```python
from build123d import *

# Parameters (mm, degrees)
BOSS_EXTRUDE1_START     = -12.7
BOSS_EXTRUDE1_OUTLINE_R = 9.525
BOSS_EXTRUDE1_DEPTH     = 12.7
SKETCH1_R               = 7.9375
BOSS_EXTRUDE2_DEPTH     = 127
BOSS_EXTRUDE3_START     = 25.4
SKETCH2_R               = 9.525
BOSS_EXTRUDE3_DEPTH     = 25.4
CHAMFER2_SIZE           = 1.5875
CUT_EXTRUDE1_DEPTH      = 166.648607751
CUT_EXTRUDE1_DEPTH_BACK = 166.648607751
SKETCH3_R               = 4.7625


# Read off the part's stored shape, not the designer's step: Boss-Extrude1
with BuildPart() as part:
    # Boss-Extrude1 outline → Boss-Extrude1 (new body)
    with BuildSketch(Plane.XY.offset(BOSS_EXTRUDE1_START)):
        Circle(BOSS_EXTRUDE1_OUTLINE_R)
    extrude(amount=BOSS_EXTRUDE1_DEPTH)

    # Sketch1 → Boss-Extrude2 (add)
    with BuildSketch(Plane(origin=(0, 0, -12.7), x_dir=(-1, 0, 0), z_dir=(0, 0, -1))):
        Circle(SKETCH1_R)
    extrude(amount=BOSS_EXTRUDE2_DEPTH)

    # Sketch2 → Boss-Extrude3 (add)
    with BuildSketch(Plane(origin=(0, 0, -139.7), x_dir=(-1, 0, 0), z_dir=(0, 0, -1)).offset(BOSS_EXTRUDE3_START)):
        Circle(SKETCH2_R)
    extrude(amount=-BOSS_EXTRUDE3_DEPTH)

    # Chamfer2
    chamfer2_edges = [part.edges().sort_by_distance(p)[0] for p in [
        (9.525, 0, -165.1),
    ]]
    chamfer(chamfer2_edges, length=CHAMFER2_SIZE)

    # Sketch3 → Cut-Extrude1 (cut, two sides: drawn at the far end of the back side and taken through both)
    with BuildSketch(Plane(origin=(0, 0, 0), x_dir=(0, 0, -1), z_dir=(1, 0, 0)).offset(-CUT_EXTRUDE1_DEPTH_BACK)):
        with Locations((152.4, 0)):
            Circle(SKETCH3_R)
    extrude(amount=CUT_EXTRUDE1_DEPTH + CUT_EXTRUDE1_DEPTH_BACK, mode=Mode.SUBTRACT)


solid = part.part
```
For this review, take the finished solid that the model builds, in its own axes (mm). A direction names the side the tool comes from. Round coordinates to 2 decimals unless told otherwise and drop trailing zeros. Write each loop counter-clockwise with the first axis right and the second up, starting at its lowest first coordinate (ties: lowest second). Pieces come first, ordered by that corner, then holes. Notation, with made-up numbers: (-7.5, 53.5) - (31.5, 53.5) arc R28 cw to (31.5, 88.5) - close; hole circle Ø4 at (8.5, 61.25). An arc over 180 degrees is marked (long way). Put each result on its own line as item: value.
Q1. We need section B-B (x = 0). Give the boundary of the cut face in (y, z) (1 decimal).
Solved:
outline: (-9.5, -163.5) - (-7.9, -165.1) - (7.9, -165.1) - (9.5, -163.5) - (9.5, -139.7) - (7.9, -139.7) - (7.9, -12.7) - (9.5, -12.7) - (9.5, 0) - (-9.5, 0) - (-9.5, -12.7) - (-7.9, -12.7) - (-7.9, -139.7) - (-9.5, -139.7) - close; hole circle Ø9.5 at (0, -152.4)
Q2. We need section A-A (y = 0). Give the boundary of the cut face in (x, z) (1 decimal), and give its area (3 significant figures).
Solved:
outline: (-9.5, -163.5) - (-7.9, -165.1) - (7.9, -165.1) - (9.5, -163.5) - (9.5, -157.2) - (-9.5, -157.2) - close; (-9.5, -147.6) - (9.5, -147.6) - (9.5, -139.7) - (7.9, -139.7) - (7.9, -12.7) - (9.5, -12.7) - (9.5, 0) - (-9.5, 0) - (-9.5, -12.7) - (-7.9, -12.7) - (-7.9, -139.7) - (-9.5, -139.7) - close
area: 2,560 mm2
Q3. Insertion check: pin 1 Ø2 at (x, z) = (2, -61.5) entering from -Y. The pin has a flat end and moves straight along its axis. Give the tip position at first contact, or say it passes through.
Solved:
pin 1: stops at y = -7.87
Q4. Mouldability with a two-part tool opening along Z and no side actions: class faces 1 (the face through (0, 0, 0)), 2 (the face through (-7.559, -5.796, -6.439)), 3 (the face through (-0.133, 4.016, -154.96)) as released by +Z, released by -Z, zero draft, split by the parting line, or undercut.
Solved:
face 1: released by +Z
face 2: zero draft
face 3: undercut
Q5. Wall thickness on probe 1 along Z at (x, y) = (-3.75, 0); probe 2 along Y at (x, z) = (-1.5, -152.4); probe 3 along Z at (x, y) = (6.5, 1): over which ranges is each line inside the solid? List them lowest first.
Solved:
probe 1: z = -165.1 to -157.16, -147.64 to 0
probe 2: y = -9.41 to -4.76, 4.76 to 9.41
probe 3: z = -165.1 to -157.06, -147.74 to 0
Q6. We need section C-C (z = -136). Give the boundary of the cut face in (x, y) (1 decimal), and give its area (3 significant figures).
Solved:
outline: circle Ø15.9 at (0, 0)
area: 198 mm2
Q7. Machinability: for faces 4 (the face through (-2, 8, -12.7)), 5 (the face through (0, 0, -165.1)), which of the approach directions +Z, -Z, +X, -X, +Y, -Y give a long, thin tool a straight path to every point of the face, cutting with its end or side? Answer none if there is none.
Solved:
face 4: none
face 5: -Z, +X, -X, +Y, -Y
